Autodesk Inventor part; units mm, degrees
ref_plane "Plano de trabajo2" through (0, 205.5279, 120) normal (1, 0, 0) x (0, 0, -1)
ref_plane "YZ Plane" through (0, 0, 0) normal (1, 0, 0) x (0, 1, 0)
ref_plane "XZ Plane" through (0, 0, 0) normal (0, 1, 0) x (-1, 0, 0)
sketch "Boceto1" plane through (0, 0, 0) normal (0, 0, 1) x (1, 0, 0)
  line L0 (0, 0) -> (70.9542, 0)
  line L1 (70.9542, 0) -> (140, -200)
  line L2 (140, -200) -> (0, -200)
  line L3 (0, -200) -> (0, 0) construction
  line L4 (0, 0) -> (-70.9542, 0)
  line L5 (-70.9542, 0) -> (-140, -200)
  line L6 (-140, -200) -> (0, -200)
  dimension "d0" = 280
  dimension "d1" = 200
extrude "Extrusión1" add sketch "Boceto1" along normal mid plane 240
sketch "Boceto2" plane through (0, 0, -120) normal (0, 0, -1) x (-1, 0, 0)
  line L0 (-63.8273, -10) -> (63.8273, -10)
  line L1 (140, -200) -> (-140, -200)
  line L2 (-63.8273, -10) -> (-129.4209, -200)
  line L3 (63.8273, -10) -> (129.4209, -200)
  line L4 (70.9542, 0) -> (-70.9542, 0)
  line L5 (140, -200) -> (70.9542, 0)
  line L6 (-70.9542, 0) -> (-140, -200)
  point P0 (0, 0)
  dimension "d4" = 10
  dimension "d7" = 10
  dimension "d8" = 10
extrude "Extrusión2" cut sketch "Boceto2" against normal blind 240 contours L0 L3 L1 L2
ref_plane "Plano de trabajo2" through (0, 205.5279, 120) normal (1, 0, 0) x (0, 0, -1)
sketch "Boceto4" plane through (0, 205.5279, 120) normal (1, 0, 0) x (0, 0, -1)
  line L0 (240, -205.5279) -> (0, -205.5279)
  line L1 (0, -205.5279) -> (-80, -405.5279)
  line L2 (-80, -405.5279) -> (-76, -405.5279)
  line L3 (0, -405.5279) -> (0, -205.5279)
  line L4 (0, -215.5279) -> (-76, -405.5279)
  line L5 (0, -215.5279) -> (0, -205.5279)
  line L6 (240, -215.5279) -> (0, -215.5279)
  line L7 (0, -215.5279) -> (0, -205.5279)
  line L8 (-80, -405.5279) -> (0, -405.5279) construction
  point P0 (120, -205.5279)
  dimension "d11" = 80
  dimension "d14" = 200
extrude "Extrusión3" add sketch "Boceto4" along normal mid plane 141.908
properties part number "chasis"
CAD build for the part. Positions are in the model's coordinates, mm. A direction names the side the tool comes from. Give positions to 0.01 mm unless a question says otherwise; leave off trailing zeros. Order: outer loops, then holes, each group sorted by start corner. A loop starts at its lowest first (then second) coordinate and runs counter-clockwise, first axis right, second up. Notation, with made-up numbers: (43.5, -32) -> (83.5, -32) arc R16 ccw to (83.5, -9) -> close; hole circle Ø10 at (71.25, 78). An arc over 180 degrees is marked (long way). Return JSON: item names as keys, results as strings.
Q1. Saw through at D-D (y = -186.5). Write the cut outline in (x, z).
Working result:
{"outline": "(-135.34, -120) -> (-124.76, -120) -> (-124.76, 120) -> (-135.34, 120) -> close; (-70.95, 190.6) -> (70.95, 190.6) -> (70.95, 194.6) -> (-70.95, 194.6) -> close; (124.76, -120) -> (135.34, -120) -> (135.34, 120) -> (124.76, 120) -> close"}
Q2. Drill centre lines: line 1 (Y direction, x = 31, z = -89); line 2 (X direction, y = -80.5, z = -37); line 3 (X direction, y = -105, z = 93.5). Where is each one in solid material? Low to high.
Working result:
{"line 1": "-10 to 0", "line 2": "-98.75 to -88.17, 88.17 to 98.75", "line 3": "-107.2 to -96.62, 96.62 to 107.2"}
Q3. Flat gauge pins, fed straight in: pin 1 (8 mm diameter, centred on x = 42, y = -167.5, fed in from -Z); pin 2 (8 mm diameter, centred on y = -36, z = 107.5, fed in from -X); pin 3 (24 mm diameter, centred on y = -72, z = 162.5, fed in from -X); pin 4 (10 mm diameter, centred on x = -7, y = -129.5, fed in from +Z). Where does each tip first touch, or does it go through?
Working result:
{"pin 1": "z = 181.4", "pin 2": "x = -84.76", "pin 3": "through", "pin 4": "z = 173.8"}
Q4. Saw through at A-A (y = -117). Write the cut outline in (x, z), then the cut area to 3 significant figures.
Working result:
{"outline": "(-111.35, -120) -> (-100.77, -120) -> (-100.77, 120) -> (-111.35, 120) -> close; (-70.95, 162.8) -> (70.95, 162.8) -> (70.95, 166.8) -> (-70.95, 166.8) -> close; (100.77, -120) -> (111.35, -120) -> (111.35, 120) -> (100.77, 120) -> close", "area": "5,650 mm²"}
Q5. Saw through at C-C (x = -38.5). Write the cut outline in (y, z).
Working result:
{"outline": "(-200, 196) -> (-10, 120) -> (-10, -120) -> (0, -120) -> (0, 120) -> (-200, 200) -> close"}
Q6. Which spindle directions (+Z, -Z, +X, -X, +Y, -Y) get a long thin tool onto all of the face, cutting with end or side? Do faces 1 (the face through (-1, -3, -120)), 2 (the face through (1, -10, -2)). Say none if no direction does.
Working result:
{"face 1": "-Z, +X, -X, +Y, -Y", "face 2": "-Z, -Y"}
Q7. Mould opens along X. For faces 3 (the face through (-0.99, -98.6, 159.44)), 4 (the face through (96.165, -103.67, -1.68)), 5 (the face through (-104.994, -98.6, -1.68)) say: pulls with the +X half, pulls with the -X half, needs draft (parallel to the pull), parting line crosses it, or undercut.
Working result:
{"face 3": "needs draft", "face 4": "undercut", "face 5": "pulls with the -X half"}
Q8. Saw through at B-B (z = 18). Write the cut outline in (x, y).
Working result:
{"outline": "(-140, -200) -> (-129.42, -200) -> (-63.83, -10) -> (63.83, -10) -> (129.42, -200) -> (140, -200) -> (70.95, 0) -> (-70.95, 0) -> close"}
